Geometry check sheet. Reference: the model listing, model coordinates, mm. A direction names the side the tool comes from. Coordinates: 2 decimals unless noted, no trailing zeros. Loops run counter-clockwise (first coordinate to the right, second up) from the corner with the lowest first, then second, coordinate; pieces in that order, holes last. Notation, with made-up numbers: M 33,-19 L 40,-19 A23 ccw 40,-10 Z; hole C 55.25,89 d1. An arc over 180 degrees is marked long. Use CSV: the item, a comma, the result in double quotes.
```python
from build123d import *

# Parameters (mm, degrees)
SKETCH_1_R      = 16.5
SKETCH_1_R_2    = 10.5
SKETCH_1_R_3    = 1.6
EXTRUDE_1_DEPTH = 4


with BuildPart() as part:
    # 草图1 → 凸台-拉伸1 (new body)
    with BuildSketch(Plane.XY):
        Circle(SKETCH_1_R)
        Circle(SKETCH_1_R_2, mode=Mode.SUBTRACT)
        with Locations((0, 13.5)):
            Circle(SKETCH_1_R_3, mode=Mode.SUBTRACT)
        with Locations((11.691342951, -6.75)):
            Circle(SKETCH_1_R_3, mode=Mode.SUBTRACT)
        with Locations((-11.691342951, -6.75)):
            Circle(SKETCH_1_R_3, mode=Mode.SUBTRACT)
        with BuildLine():
            ThreePointArc((-4.331175309, 11.083813443), (-3.423257577, 13.156416973), (-5.495861107, 14.064334705))
            ThreePointArc((-5.495861107, 14.064334705), (-13.076983597, 7.55), (-14.928001695, -2.272612018))
            ThreePointArc((-14.928001695, -2.272612018), (-13.10542011, -3.613580461), (-11.764451667, -1.790998875))
            ThreePointArc((-11.764451667, -1.790998875), (-10.305702305, 5.95), (-4.331175309, 11.083813443))
        make_face(mode=Mode.SUBTRACT)
        with BuildLine():
            ThreePointArc((11.764451667, -1.790998876), (13.10542011, -3.613580461), (14.928001695, -2.272612019))
            ThreePointArc((14.928001695, -2.272612019), (13.076983597, 7.55), (5.495861107, 14.064334705))
            ThreePointArc((5.495861107, 14.064334705), (3.423257577, 13.156416973), (4.331175309, 11.083813443))
            ThreePointArc((4.331175309, 11.083813443), (10.305702305, 5.95), (11.764451667, -1.790998876))
        make_face(mode=Mode.SUBTRACT)
        with BuildLine():
            ThreePointArc((-7.433276358, -9.292814568), (-9.682162533, -9.542836512), (-9.432140589, -11.791722687))
            ThreePointArc((-9.432140589, -11.791722687), (0, -15.1), (9.432140588, -11.791722687))
            ThreePointArc((9.432140588, -11.791722687), (9.682162533, -9.542836512), (7.433276358, -9.292814568))
            ThreePointArc((7.433276358, -9.292814568), (0, -11.9), (-7.433276358, -9.292814568))
        make_face(mode=Mode.SUBTRACT)
    extrude(amount=EXTRUDE_1_DEPTH)


solid = part.part
```
1. Set-up check for faces 1 (the cylindrical face through (-13.005, 7.673, 1.972)), 2 (the flat face through (-4, 10, 4)): record each of +Z, -Z, +X, -X, +Y, -Y from which the full face is reachable in a straight line by a thin tool's end or side.
The answers:
face 1,"+Z, -Z"
face 2,"+Z, +X, -X, +Y, -Y"
2. Section check C-C, the plane z = 0.9. Record the cut outline in (x, y).
The answers:
outline,"C 0,0 d33; hole M -14.93,-2.27 A1.6 ccw -11.76,-1.79 A11.9 cw -4.33,11.08 A1.6 ccw -5.5,14.06 A15.1 ccw Z; hole C -11.69,-6.75 d3.2; hole C 0,0 d21; hole M -9.43,-11.79 A15.1 ccw 9.43,-11.79 A1.6 ccw 7.43,-9.29 A11.9 cw -7.43,-9.29 A1.6 ccw Z; hole C 0,13.5 d3.2; hole M 4.33,11.08 A11.9 cw 11.76,-1.79 A1.6 ccw 14.93,-2.27 A15.1 ccw 5.5,14.06 A1.6 ccw Z; hole C 11.69,-6.75 d3.2"
3. Thickness scan on line 1 (Y direction, x = 0, z = 2.25); line 2 (Y direction, x = -7, z = 3.7); line 3 (X direction, y = 1, z = 2.1). Record the ranges inside material, lowest first. Write a range as [from, to].
The answers:
line 1,"[-16.5, -15.1], [-11.9, -10.5], [10.5, 11.9], [15.1, 16.5]"
line 2,"[-14.94, -13.38], [-9.62, -7.83], [7.83, 9.62], [13.38, 14.94]"
line 3,"[-16.47, -15.07], [-11.86, -10.45], [10.45, 11.86], [15.07, 16.47]"
4. Section check A-A, the plane y = 0. Record the cut outline in (x, z).
The answers:
outline,"M -16.5,0 L -15.1,0 L -15.1,4 L -16.5,4 Z; M -11.9,0 L -10.5,0 L -10.5,4 L -11.9,4 Z; M 10.5,0 L 11.9,0 L 11.9,4 L 10.5,4 Z; M 15.1,0 L 16.5,0 L 16.5,4 L 15.1,4 Z"
5. Gauge pin test, flat ends, axial feed: P1, Ø2, axis at y = 3, z = 2.5, coming from the -X side; P2, Ø1.5, axis at y = 6, z = 3, coming from the -X side; P3, Ø2.5, axis at x = 11.69, y = -6.75, coming from the +Z side; P4, Ø1.5, axis at x = 9, z = 3.5, coming from the +Y side. Record the tip position at first contact, or that the pin passes through.
The answers:
P1,"x = -16.38"
P2,"x = -15.64"
P3,"through"
P4,"y = 14.29"
